Could you check a few things on this model? Use its own coordinates, in mm. Round coordinates to 2 decimals unless told otherwise and drop trailing zeros. Write each loop counter-clockwise with the first axis right and the second up, starting at its lowest first coordinate (ties: lowest second). Pieces come first, ordered by that corner, then holes. Notation, with made-up numbers: (73, 23.5) - (82, 23.5) arc R21 cw to (82, 51.5) - close; hole circle Ø11 at (22, -38). An arc over 180 degrees is marked (long way). Write each question's results on one line, items separated by ' | '. Start each with the question number.
(1) Imagine slicing it at B-B on y = -186. Write out the boundary of the cut face in (x, z).
(2) Imagine slicing it at A-A on z = 0.75. Write out the boundary of the cut face in (x, y).
(3) Please list where this line runs through material, in increasing order: line 1 (X direction, y = -206.5, z = 1.35). Write a range as [from, to].
Autodesk Inventor part; units mm, degrees
ref_plane "YZ Plane" through (0, 0, 0) normal (1, 0, 0) x (0, 1, 0)
ref_plane "XZ Plane" through (0, 0, 0) normal (0, 1, 0) x (-1, 0, 0)
ref_plane "XY Plane" through (0, 0, 0) normal (0, 0, 1) x (1, 0, 0)
sketch "Sketch1" plane through (0, 0, 0) normal (0, 0, 1) x (1, 0, 0)
  line L0 (-244.5, 244.5) -> (244.5, 244.5)
  line L1 (244.5, 244.5) -> (244.5, -244.5)
  line L2 (244.5, -244.5) -> (-244.5, -244.5)
  line L3 (-244.5, -244.5) -> (-244.5, 244.5)
  line L4 (-244.5, 244.5) -> (244.5, -244.5) construction
  line L5 (244.5, 244.5) -> (-244.5, -244.5) construction
  line L6 (-229.5, -229.5) -> (229.5, -229.5)
  line L7 (229.5, -229.5) -> (229.5, 229.5)
  line L8 (229.5, 229.5) -> (-229.5, 229.5)
  line L9 (-229.5, 229.5) -> (-229.5, -229.5)
  line L10 (-229.5, -229.5) -> (229.5, 229.5) construction
  line L11 (229.5, -229.5) -> (-229.5, 229.5) construction
  line L12 (-229.5, 229.5) -> (-244.5, 244.5)
  line L13 (229.5, -229.5) -> (244.5, -244.5)
  point P0 (0, 0)
  dimension "d1" = 489
  dimension "d18" = 15
  dimension "d19" = 489
extrude "Plate1" add sketch "Sketch1" along normal blind 2 contours L0 L1 L13 L7 L8 L12
chamfer "Corner Chamfer1" distance 1 angle 45 2 edges at (-244.5, 244.5, 1) (244.5, -244.5, 1)
equation "\"d19\" = d1"
equation "\"d3\" = Thickness"
equation "\"BendRadius\" = Thickness"
equation "\"BendReliefWidth\" = Thickness"
equation "\"BendReliefDepth\" = 0.5 * Thickness"
equation "\"CornerReliefSize\" = 4 * Thickness"
equation "\"MinimumRemnant\" = 2 * Thickness"
equation "\"TransitionRadius\" = BendRadius"
equation "\"JacobiRadiusSize\" = BendRadius"
equation "\"GapSize\" = Thickness"
properties part number "PNS waste water bin 06"
Response:
1) outline: (229.5, 0) - (244.5, 0) - (244.5, 2) - (229.5, 2) - close
2) outline: (-243.79, 243.79) - (-229.5, 229.5) - (229.5, 229.5) - (229.5, -229.5) - (243.79, -243.79) - (244.5, -243.5) - (244.5, 244.5) - (-243.5, 244.5) - close
3) line 1: [229.5, 244.5]
